Part model, mm, in its own coordinate system. A direction names the side the tool comes from. Give positions to 0.01 mm unless a question says otherwise; leave off trailing zeros. Write each loop counter-clockwise with the first axis right and the second up, starting at its lowest first coordinate (ties: lowest second). Pieces come first, ordered by that corner, then holes. Notation, with made-up numbers: (60.25, 17) - (108.25, 17) arc R25 cw to (108.25, 30) - close; hole circle Ø8 at (-10, 79.25). An arc over 180 degrees is marked (long way). Answer in a Markdown table with one row per item. Add a question column.
1. Band-saw the part on D-D on x = 2.05. Write the cut outline in (y, z), plus the area to 3 significant figures.
2. Drop flat-ended pins along their axis: pin 1 Ø0.6 at (x, y) = (1.5, 10) entering from +Z; pin 2 Ø0.5 at (y, z) = (-5, -0.5) entering from -X; pin 3 Ø0.5 at (y, z) = (-2.5, -0.5) entering from +X. Give the stop position or say it passes through.
3. Probe line 1 along Z through (x, y) = (0.85, 6.5); line 2 along X through (y, z) = (6, 0.95); line 3 along Y through (x, z) = (-0.6, -1.15). List the from-to ranges inside material, lowest first.
4. Band-saw the part on C-C on y = -2.5. Write the cut outline in (x, z), plus the area to 3 significant figures.
5. Band-saw the part on B-B on x = -0.95. Write the cut outline in (y, z).
6. Which spindle directions (+Z, -Z, +X, -X, +Y, -Y) get a long thin tool onto all of the face, cutting with end or side? Do faces 1 (the cylindrical face through (2.215, -3.451, 0.699)), 2 (the flat face through (-2.5, -3.5, -0.5)), 3 (the flat face through (0, 5.5, 1.2)), 4 (the flat face through (0, 7, -2)), 5 (the cylindrical face through (-2.199, -3.451, 0.715)). Say none if no direction does.
```python
from build123d import *

# Parameters (mm, degrees)
F1_DEPTH = 7
F2_W     = 6
F2_H     = 5
F3_DEPTH = 5.5
F4_W     = 6
F4_H     = 3
F5_DEPTH = 3
F6_W     = 6
F6_H     = 2
F7_DEPTH = 2
F9_DEPTH = 1
F10_SIZE = 0.99999


# Not quite as in the source:
# - a fillet or chamfer is up to 0.001 mm smaller than in the source, because OpenCascade refuses the exact size


with BuildPart() as f1:
    # F0 (on Front) → F1 (new body)
    with BuildSketch(Plane.XZ):
        with BuildLine():
            Line((-2.5, -1), (2.5, -1))
            Line((2.5, -1), (2.5, 0))
            ThreePointArc((2.5, 0), (2.2071067812, 0.7071067812), (1.5, 1))
            Line((1.5, 1), (-1.5, 1))
            ThreePointArc((-1.5, 1), (-2.2071067812, 0.7071067812), (-2.5, 0))
            Line((-2.5, 0), (-2.5, -1))
        make_face()
    extrude(amount=F1_DEPTH)

    # F2 (on face) → F3 (join)
    with BuildSketch(Plane(origin=(0, 0, 0), x_dir=(-1, 0, 0), z_dir=(0, 1, 0))):
        with Locations((0, -0.5)):
            Rectangle(F2_W, F2_H)
        with BuildLine():
            ThreePointArc((1.5, 1), (2.2071067812, 0.7071067812), (2.5, 0))
            Line((2.5, 0), (2.5, -1))
            Line((2.5, -1), (-2.5, -1))
            Line((-2.5, -1), (-2.5, 0))
            ThreePointArc((-2.5, 0), (-2.2071067812, 0.7071067812), (-1.5, 1))
            Line((-1.5, 1), (1.5, 1))
        make_face(mode=Mode.SUBTRACT)
        with BuildLine():
            Line((2.5, -1), (2.5, 0))
            ThreePointArc((2.5, 0), (2.2071067812, 0.7071067812), (1.5, 1))
            Line((1.5, 1), (-1.5, 1))
            ThreePointArc((-1.5, 1), (-2.2071067812, 0.7071067812), (-2.5, 0))
            Line((-2.5, 0), (-2.5, -1))
            Line((-2.5, -1), (2.5, -1))
        make_face()
    extrude(amount=F3_DEPTH)

    # F4 (on face) → F5 (join)
    with BuildSketch(Plane(origin=(0, 5.5, 0), x_dir=(-1, 0, 0), z_dir=(0, 1, 0))):
        with Locations((0, -0.5)):
            Rectangle(F4_W, F4_H)
    extrude(amount=F5_DEPTH)

    # F6 (on face) → F7 (join)
    with BuildSketch(Plane(origin=(0, 8.5, 0), x_dir=(-1, 0, 0), z_dir=(0, 1, 0))):
        with Locations((0, -0.5)):
            Rectangle(F6_W, F6_H)
    extrude(amount=F7_DEPTH)

    # F8 (on face) → F9 (cut)
    with BuildSketch(Plane(origin=(-3, 0, 0), x_dir=(0, -1, 0), z_dir=(-1, 0, 0))):
        Polygon((-5.5, -2), (-5.5, 1), (-8.5, 1), (-8.5, 0.5), (-10.5, 0.5), (-10.5, -1.5), (-8.5, -1.5), (-8.5, -2), align=None)
    extrude(amount=-F9_DEPTH, mode=Mode.SUBTRACT)

    # F10 (size 1 in the source; OpenCascade refuses exactly that, so slightly less here)
    f10_edges = [f1.edges().sort_by_distance(p)[0] for p in [
        (-2, 5.5, -0.5),
    ]]
    chamfer(f10_edges, length=F10_SIZE)


solid = f1.part
```
Values:
| question | item | result |
|---|---|---|
| 1 | outline | (-7, -1) - (0, -1) - (0, -3) - (5.5, -3) - (5.5, -2) - (8.5, -2) - (8.5, -1.5) - (10.5, -1.5) - (10.5, 0.5) - (8.5, 0.5) - (8.5, 1) - (5.5, 1) - (5.5, 2) - (0, 2) - (0, 0.84) - (-7, 0.84) - close |
| 1 | area | 53.3 mm² |
| 2 | pin 1 | stops at z = 0.5 |
| 2 | pin 2 | stops at x = -2.5 |
| 2 | pin 3 | stops at x = 2.5 |
| 3 | line 1 | z = -2 to 1 |
| 3 | line 2 | x = -2.5 to 3 |
| 3 | line 3 | y = 0 to 10.5 |
| 4 | outline | (-2.5, -1) - (2.5, -1) - (2.5, 0) arc R1 ccw to (1.5, 1) - (-1.5, 1) arc R1 ccw to (-2.5, 0) - close |
| 4 | area | 9.57 mm² |
| 5 | outline | (-7, -1) - (0, -1) - (0, -3) - (5.5, -3) - (5.5, -2) - (8.5, -2) - (8.5, -1.5) - (10.5, -1.5) - (10.5, 0.5) - (8.5, 0.5) - (8.5, 1) - (5.5, 1) - (5.5, 2) - (0, 2) - (0, 1) - (-7, 1) - close |
| 6 | face 1 | +Z, +X, -Y |
| 6 | face 2 | +Z, -Z, -X, -Y |
| 6 | face 3 | +Z, +X, -X, +Y |
| 6 | face 4 | -Z, +X, -X, +Y |
| 6 | face 5 | +Z, -X, -Y |
